```python
from build123d import *

# Parameters (mm, degrees)
SKETCH1_W           = 100
SKETCH1_H           = 80
SKETCH1_R           = 1.651
BOSS_EXTRUDE1_DEPTH = 2.032
FILLET1_R           = 2.54
FILLET2_R           = 2.54


with BuildPart() as part:
    # Sketch1 → Boss-Extrude1 (new body)
    with BuildSketch(Plane(origin=(0, 0, 0), x_dir=(1, 0, 0), z_dir=(0, 1, 0))):
        with Locations((3.469387755, -11.530612245)):
            Rectangle(SKETCH1_W, SKETCH1_H)
        with Locations(Location((-36.530612245, 18.469387755, 0), (0, 0, 270))):
            Circle(SKETCH1_R, mode=Mode.SUBTRACT)
        with Locations(Location((-36.530612245, -41.530612245, 0), (0, 0, 270))):
            Circle(SKETCH1_R, mode=Mode.SUBTRACT)
        with Locations(Location((-16.530612245, 21.469387755, 0), (0, 0, 270))):
            Circle(SKETCH1_R, mode=Mode.SUBTRACT)
        with Locations(Location((23.469387755, 21.469387755, 0), (0, 0, 270))):
            Circle(SKETCH1_R, mode=Mode.SUBTRACT)
        with Locations(Location((-16.530612245, -18.530612245, 0), (0, 0, 270))):
            Circle(SKETCH1_R, mode=Mode.SUBTRACT)
        with Locations(Location((23.469387755, -18.530612245, 0), (0, 0, 270))):
            Circle(SKETCH1_R, mode=Mode.SUBTRACT)
        with Locations(Location((-17.39026229, 9.3290378, 0), (0, 0, 270))):
            Circle(SKETCH1_R, mode=Mode.SUBTRACT)
        with Locations(Location((24.3290378, 9.3290378, 0), (0, 0, 270))):
            Circle(SKETCH1_R, mode=Mode.SUBTRACT)
        with Locations(Location((43.469387755, -41.530612245, 0), (0, 0, 90))):
            Circle(SKETCH1_R, mode=Mode.SUBTRACT)
        with Locations(Location((43.469387755, 18.469387755, 0), (0, 0, 90))):
            Circle(SKETCH1_R, mode=Mode.SUBTRACT)
        with Locations(Location((-17.39026229, -32.39026229, 0), (0, 0, 270))):
            Circle(SKETCH1_R, mode=Mode.SUBTRACT)
        with Locations(Location((24.3290378, -32.39026229, 0), (0, 0, 270))):
            Circle(SKETCH1_R, mode=Mode.SUBTRACT)
    extrude(amount=BOSS_EXTRUDE1_DEPTH)

    # Fillet1
    fillet1_edges = [part.edges().sort_by_distance(p)[0] for p in [
        (-46.530612245, 1.016, 51.530612245),
    ]]
    fillet(fillet1_edges, radius=FILLET1_R)

    # Fillet2
    fillet2_edges = [part.edges().sort_by_distance(p)[0] for p in [
        (-46.530612245, 1.016, -28.469387755),
        (53.469387755, 1.016, -28.469387755),
        (53.469387755, 1.016, 51.530612245),
    ]]
    fillet(fillet2_edges, radius=FILLET2_R)


solid = part.part
```
Design review of the part built by this model. Coordinates are the model's own, in mm. Give positions to 0.01 mm unless a question says otherwise; leave off trailing zeros. Order: outer loops, then holes, each group sorted by start corner. A loop starts at its lowest first (then second) coordinate and runs counter-clockwise, first axis right, second up. Notation, with made-up numbers: (68, 82) -> (111, 82) arc R27 cw to (111, 105) -> close; hole circle Ø8 at (1, -31). An arc over 180 degrees is marked (long way). Write item = value, one per line. Start each with the question number.
(1) Mouldability with a two-part tool opening along X and no side actions: class faces 1 (the face through (-46.531, 1, 12)), 2 (the face through (52.706, 1.03, -27.745)), 3 (the face through (-16.035, 1.002, -19.895)) as +X half, -X half, draft (parallel to the pull), parting line (faces both ways), or undercut.
(2) We need section A-A on z = -22. Write out the cut boundary in (x, y), plus the area to 3 significant figures.
(3) For pin 1 (5.5 mm diameter, centred on x = -36.53, z = 41.53, fed in from -Y), flat-tipped, find the tip position at first contact; note if it passes through.
Numbers:
q1.face_1 = -X half
q1.face_2 = +X half
q1.face_3 = undercut
q2.outline = (-46.53, 0) -> (-18.09, 0) -> (-18.09, 2.03) -> (-46.53, 2.03) -> close; (-14.97, 0) -> (21.91, 0) -> (21.91, 2.03) -> (-14.97, 2.03) -> close; (25.03, 0) -> (53.47, 0) -> (53.47, 2.03) -> (25.03, 2.03) -> close
q2.area = 190 mm^2
q3.pin_1 = 0
